For this review, take the finished solid that the model builds, in its own axes (mm). Coordinates: 2 decimals unless noted, no trailing zeros. Loops run counter-clockwise (first coordinate to the right, second up) from the corner with the lowest first, then second, coordinate; pieces in that order, holes last. Notation, with made-up numbers: (-26.5, 62) - (31.5, 62) arc R19 cw to (31.5, 73) - close; hole circle Ø11 at (53, 40). An arc over 180 degrees is marked (long way). Answer as a JSON object with one key per item and string values. Group by question number.
Item 1: To check wall thickness, follow line 1 (X direction, y = -9.5, z = 8.75); line 2 (X direction, y = -15.5, z = 9); line 3 (Y direction, x = 7, z = 5.25). State the ranges of each line that lie inside material, in increasing order.
Item 2: We need section A-A (x = -17.5). Give the boundary of the cut face in (y, z), then the cut area to 3 significant figures.
Item 3: We need section C-C (x = -50). Give the boundary of the cut face in (y, z).
Item 4: Clearance check with flat-ended pins moving along their axes: pin 1 (1.5 mm diameter, centred on y = -9, z = 6.5, fed in from +X); pin 2 (13 mm diameter, centred on x = 91.28, y = -15, fed in from -Z). State where each tip first meets the part, or that it passes through.
Item 5: We need section B-B (y = -15). Give the boundary of the cut face in (x, z).
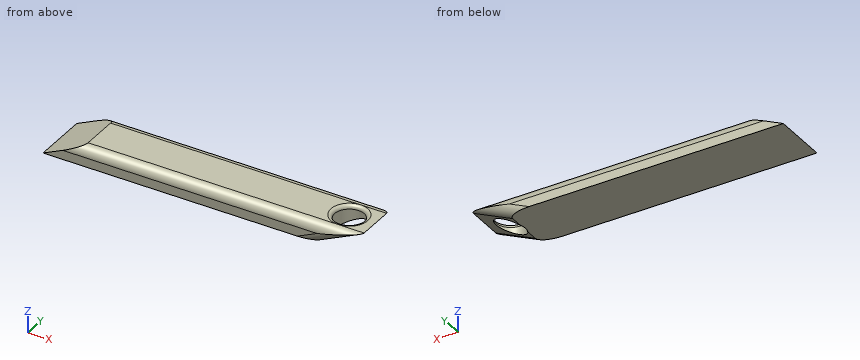
from build123d import *

# Parameters (mm, degrees)
F1_DEPTH = 30
F2_R     = 8
F3_DEPTH = 25
F4_R     = 5
F5_R     = 1.99999


# Not quite as in the source:
# - a fillet or chamfer is up to 0.001 mm smaller than in the source, because OpenCascade refuses the exact size


with BuildPart() as f1:
    # F0 (on Front) → F1 (new body)
    with BuildSketch(Plane.XZ):
        Polygon((-44.6024514475, 10), (-66.0475206525, 0), (83.9524793475, 0), (105.3975485525, 10), align=None)
    extrude(amount=F1_DEPTH)

    # F2 (on Top) → F3 (cut)
    with BuildSketch(Plane.XY):
        with Locations((91.2811756134, -15)):
            Circle(F2_R)
    extrude(amount=F3_DEPTH, mode=Mode.SUBTRACT)

    # F4
    f4_edges = [f1.edges().sort_by_distance(p)[0] for p in [
        (30.397549, 0, 10),
        (30.397549, -30, 10),
        (94.675014, -30, 5),
        (94.675014, 0, 5),
    ]]
    fillet(f4_edges, radius=F4_R)

    # F5 (radius 2 in the source; OpenCascade refuses exactly that, so slightly less here)
    f5_edges = [f1.edges().sort_by_distance(p)[0] for p in [
        (83.281176, -15, 10),
    ]]
    fillet(f5_edges, radius=F5_R)


solid = f1.part
Check sheet entries:
{
 "1": {"line 1": "x = -47.28 to 85.27, 97.29 to 102.72", "line 2": "x = -46.75 to 83.03, 99.53 to 103.25", "line 3": "y = -29.99 to -0.01"},
 "2": {"outline": "(-30, 0) - (0, 0) - (0, 5) arc R5 ccw to (-5, 10) - (-25, 10) arc R5 ccw to (-30, 5) - close", "area": "289 mm2"},
 "3": {"outline": "(-30, 0) - (0, 0) - (0, 5) arc R5 ccw to (-0.66, 7.48) - (-29.34, 7.48) arc R5 ccw to (-30, 5) - close"},
 "4": {"pin 1": "stops at x = 99.5", "pin 2": "passes through"},
 "5": {"outline": "(-66.05, 0) - (83.28, 0) - (83.28, 8) arc R2 ccw to (81.28, 10) - (-44.6, 10) - close; (99.28, 7.15) - (105.4, 10) - (101.28, 10) arc R2 ccw to (99.28, 8) - close"}
}
